from build123d import *

# Parameters (mm, degrees)
SKETCH2_W             = 30
SKETCH2_H             = 130
BOSS_EXTRUDE1_DEPTH   = 10
M3X0_5_TAPPED_HOLE2_D = 2.5
CUT_EXTRUDE3_DEPTH    = 75.64013832
FILLET3_RADIUS        = 8
FILLET3_LENGTH        = 10
FILLET4_R             = 4
M3X0_5_TAPPED_HOLE3_D = 2.5


with BuildPart() as part:
    # Sketch2 → Boss-Extrude1 (new body)
    with BuildSketch(Plane.XY):
        with Locations((-14.802371542, -2.697628458)):
            Rectangle(SKETCH2_W, SKETCH2_H)
    extrude(amount=BOSS_EXTRUDE1_DEPTH)

    # M3x0.5 Tapped Hole2 (through all)
    with Locations(Plane.XY.offset(10)):
        with Locations((-14.802371542, 35.302371542), (-21.802371542, 42.302371542), (-14.802371542, 49.302371542), (-7.802371542, 42.302371542)):
            Hole(M3X0_5_TAPPED_HOLE2_D / 2)

    # Sketch6 → Cut-Extrude3 (cut, through all)
    with BuildSketch(Plane.XY.offset(10)):
        Polygon((-29.802371542, -67.697628458), (-22.802371542, -67.697628458), (-22.802371542, -33.848814229), (-29.802371542, 0), align=None)
        Polygon((0.197628458, -67.697628458), (-6.802371542, -67.697628458), (-6.802371542, -33.848814229), (0.197628458, 0), align=None)
    extrude(amount=-CUT_EXTRUDE3_DEPTH, mode=Mode.SUBTRACT)

    # Fillet3: full round fillet: the end face becomes a half cylinder, R = half its width
    fillet3_face = Plane((-14.802371542, -67.697628458, 5), x_dir=(0, 0, 1), z_dir=(0, -1, 0))  # on the end face: x along it, z out of the body
    fillet3_slab = fillet3_face.offset(-FILLET3_RADIUS / 2) * Box(FILLET3_LENGTH, 2 * FILLET3_RADIUS, FILLET3_RADIUS, mode=Mode.PRIVATE)  # the body's end, R deep
    fillet3_round = Plane((-14.802371542, -59.697628458, 5), x_dir=(0, -1, 0), z_dir=(0, 0, 1)) * Cylinder(FILLET3_RADIUS, FILLET3_LENGTH, mode=Mode.PRIVATE)  # its axis R under the face
    add(fillet3_slab - fillet3_round, mode=Mode.SUBTRACT)

    # Fillet4
    fillet4_edges = [part.edges().sort_by_distance(p)[0] for p in [
        (0.197628458, 31.151185771, 0),
        (0.197628458, 31.151185771, 10),
        (-3.302371542, -16.924407115, 10),
        (-6.802371542, -33.848814229, 5),
        (0.197628458, 0, 5),
        (-3.302371542, -16.924407115, 0),
        (-29.802371542, 31.151185771, 10),
        (-26.302371542, -16.924407115, 10),
        (-29.802371542, 0, 5),
        (-22.802371542, -33.848814229, 5),
        (-26.302371542, -16.924407115, 0),
        (-29.802371542, 31.151185771, 0),
        (-22.802371542, -46.773221344, 10),
        (-22.802371542, -46.773221344, 0),
        (-6.802371542, -46.773221344, 10),
        (-6.802371542, -46.773221344, 0),
        (-14.802371542, -67.697628458, 0),
        (-14.802371542, -67.697628458, 10),
        (-29.802371542, 62.302371542, 5),
        (0.197628458, 62.302371542, 5),
    ]]
    fillet(fillet4_edges, radius=FILLET4_R)

    # M3x0.5 Tapped Hole3 (through all)
    with Locations(Plane.XY.offset(10)):
        with Locations((-14.802371542, 42.302371542)):
            Hole(M3X0_5_TAPPED_HOLE3_D / 2)


solid = part.part
For this review, take the finished solid that the model builds, in its own axes (mm). A direction names the side the tool comes from. Round coordinates to 2 decimals unless told otherwise and drop trailing zeros. Write each loop counter-clockwise with the first axis right and the second up, starting at its lowest first coordinate (ties: lowest second). Pieces come first, ordered by that corner, then holes. Notation, with made-up numbers: M -7,16 L 9,16 A36 ccw 9,54 Z; hole C 84.5,49.25 d11. An arc over 180 degrees is marked long. Write item = value, one per line. Start each with the question number.
(1) The part is to be moulded in two halves that separate along Y. For faces 1 (the face through (-4.372, -16.462, 1.203)), 2 (the face through (-8.379, 41.193, 4.93)), 3 (the face through (-0.943, 31.789, 1.203)), say which applies: +Y half, -Y half, draft (parallel to the pull), parting line (faces both ways), or undercut.
(2) For line 1 along Y through (x, z) = (-15, 5.5); line 2 along X through (y, z) = (35.5, 1.25); line 3 along X through (y, z) = (-51, 4), list the stretches that pass through material, from the lowest coordinate up.
(3) We need section A-A (y = -55). Give the boundary of the cut face in (x, z).
(4) For faces 4 (the face through (-21.66, -46.8, 8.8)), 5 (the face through (-7.943, -47.156, 1.203)), 6 (the face through (-28.133, 61.554, 5.07)), 7 (the face through (-21.66, -46.8, 1.2)), list the 3-axis set-ups (+Z, -Z, +X, -X, +Y, -Y) from which the entire face can be reached by the end or side of a thin tool; tool diameter is ignored.
(5) Clearance check with flat-ended pins moving along their axes: pin 1 Ø2 at (y, z) = (15, 7.5) entering from +X; pin 2 Ø1.5 at (x, y) = (-21.8, 42.3) entering from -Z; pin 3 Ø0.6 at (y, z) = (-47, 5.5) entering from -X; pin 4 Ø2 at (y, z) = (-42.5, 5) entering from +X. State where each tip first meets the part, or that it passes through.
(6) We need section B-B (z = 1.5). Give the number of separate pieces and of enclosed holes in the cut face, then the cut area to 3 significant figures.
(7) We need section C-C (y = 4). Give the boundary of the cut face in (x, z).
Results found:
q1.face_1 = -Y half
q1.face_2 = undercut
q1.face_3 = draft
q2.line_1 = -67.7 to 34.07, 36.54 to 41.07, 43.54 to 48.07, 50.54 to 62.3
q2.line_2 = -28.71 to -16.04, -13.57 to -0.9
q2.line_3 = -22.8 to -6.8
q3.outline = M -22.8,4 A4 ccw -18.8,0 L -10.8,0 A4 ccw -6.8,4 L -6.8,6 A4 ccw -10.8,10 L -18.8,10 A4 ccw -22.8,6 Z
q4.face_4 = +Z, -X, -Y
q4.face_5 = -Z, +X, -Y
q4.face_6 = +Z, -Z, -X, +Y
q4.face_7 = -Z, -X, -Y
q5.pin_1 = 0.17
q5.pin_2 = through
q5.pin_3 = -22.8
q5.pin_4 = -6.8
q6.separate_pieces = 1
q6.enclosed_holes = 5
q6.area = 2,900 mm²
q7.outline = M -29.8,4 A4 ccw -25.8,0 L -3.8,0 A4 ccw 0.2,4 L 0.2,6 A4 ccw -3.8,10 L -25.8,10 A4 ccw -29.8,6 Z
